Can you work these out from the model? Positions are in its coordinate system, mm. Face numbers are marked on the shaded views. A direction names the side the tool comes from. Round coordinates to 2 decimals unless told otherwise and drop trailing zeros. Order: outer loops, then holes, each group sorted by start corner. A loop starts at its lowest first (then second) coordinate and runs counter-clockwise, first axis right, second up.
Q1. If we section it at A-A (z = 17.75): Please give me the cut outline in (x, y) (3 decimals).
Q2. Will these pins go through, and if not, where does the flat tip stop? P1, Ø2, axis at x = 3, y = -6, coming from the +Z side; P2, Ø1.6, axis at x = 6, z = 19.5, coming from the -Y side; P3, Ø6, axis at x = -2, y = 1, coming from the +Z side.
Q3. We'd pull the mould along Y, two halves only. Please class the marked faces 4, 5 and 6: pulls with the +Y half, pulls with the -Y half, needs draft (parallel to the pull), parting line crosses it, or undercut.
Q4. If I drill on line 1 (Y direction, x = 0, z = 7.75) (3 decimals); line 2 (Z direction, x = 4.5, y = -5.75); line 3 (Y direction, x = -3.75, z = 5.25), over which ranges is the centre line in solid material (lowest first)?
Q5. For the marked faces 1, 2 and 3, which set-ups out of +Z, -Z, +X, -X, +Y, -Y let a thin tool reach every point of the face, with its end or its side?
Q6. If we section it at C-C (x = 6.5): Please give me the cut outline in (y, z).
Q7. If we section it at D-D (y = -2.75): Please give me the cut outline in (x, z) (3 decimals).
Q8. If we section it at B-B (z = 11.5): Please give me the cut outline in (x, y) (1 decimal), plus the area to 3 significant figures.
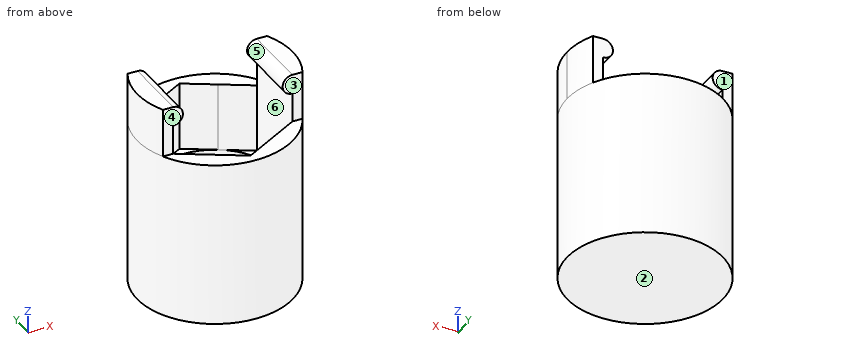
from build123d import *

# Parameters (mm, degrees)
F0_R      = 6.125
F1_DEPTH  = 2
F0_R_2    = 8
F2_DEPTH  = 10
F3_R      = 8
F4_DEPTH  = 7
F6_DEPTH  = 5
F8_DEPTH  = 7.0725407976
F10_DEPTH = 7.0725407976


with BuildPart() as f1:
    # F0 (on Top) → F1 (new body)
    with BuildSketch(Plane.XY):
        Circle(F0_R)
    extrude(amount=F1_DEPTH)

    # F0 (on Top) → F2 (join)
    with BuildSketch(Plane.XY):
        Circle(F0_R_2)
        Circle(F0_R, mode=Mode.SUBTRACT)
    extrude(amount=F2_DEPTH)

    # F3 (on face) → F4 (join)
    with BuildSketch(Plane.XY.offset(10)):
        Circle(F3_R)
        Polygon((3.0624998551, 5.3044056818), (6.125, 3.5362703988), (6.125, 0), (6.125, -3.5362703988), (3.0625000444, -5.3044055725), (0, -7.0725407976), (-3.0625000444, -5.3044055725), (-6.125, -3.5362703988), (-6.125, 0), (-6.125, 3.5362703988), (-3.0624999859, 5.3044056063), (0, 7.0725407976), align=None, mode=Mode.SUBTRACT)
    extrude(amount=F4_DEPTH)

    # F5 (on face) → F6 (join)
    with BuildSketch(Plane.XY.offset(17)):
        with BuildLine():
            Line((-6.125, -3.5362703988), (-6.125, 3.5362703988))
            Line((-6.125, 3.5362703988), (-7.1759871563, 3.5362703988))
            ThreePointArc((-7.1759871563, 3.5362703988), (-8, 0), (-7.1759871563, -3.5362703988))
            Line((-7.1759871563, -3.5362703988), (-6.125, -3.5362703988))
        make_face()
        with BuildLine():
            ThreePointArc((8, 0), (7.7912738769, 1.8155030639), (7.1759871563, 3.5362703988))
            Line((7.1759871563, 3.5362703988), (6.125, 3.5362703988))
            Line((6.125, 3.5362703988), (6.125, -3.5362703988))
            Line((6.125, -3.5362703988), (7.1759871563, -3.5362703988))
            ThreePointArc((7.1759871563, -3.5362703988), (7.7912738769, -1.8155030639), (8, 0))
        make_face()
    extrude(amount=F6_DEPTH)

    # F7 (on face) → F8 (join, through all)
    with BuildSketch(Plane(origin=(0, 3.5362703988, 0), x_dir=(-1, 0, 0), z_dir=(0, 1, 0))):
        with BuildLine():
            Line((6.125, 20), (6.125, 22))
            ThreePointArc((6.125, 22), (5.125, 21), (6.125, 20))
        make_face()
    extrude(amount=-F8_DEPTH)

    # F9 (on face) → F10 (join, through all)
    with BuildSketch(Plane(origin=(0, 3.5362703988, 0), x_dir=(-1, 0, 0), z_dir=(0, 1, 0))):
        with BuildLine():
            Line((-6.125, 22), (-6.125, 20))
            ThreePointArc((-6.125, 20), (-5.125, 21), (-6.125, 22))
        make_face()
    extrude(amount=-F10_DEPTH)


solid = f1.part
Solution:
1. outline: (-7.176, -3.536) - (-6.125, -3.536) - (-6.125, 3.536) - (-7.176, 3.536) arc R8 ccw to start; (6.125, -3.536) - (7.176, -3.536) arc R8 ccw to (7.176, 3.536) - (6.125, 3.536) - close
2. P1: stops at z = 17
2. P2: stops at y = -3.54
2. P3: stops at z = 2
3. face 4: pulls with the -Y half
3. face 5: needs draft
3. face 6: undercut
4. line 1: y = -8 to -6.125, 6.125 to 8
4. line 2: z = 0 to 17
4. line 3: y = -7.07 to -4.84, 4.84 to 7.07
5. face 1: +Z, +X, -X, +Y
5. face 2: -Z, +X, -X, +Y, -Y
5. face 3: +Z, +X, -X, -Y
6. outline: (-4.66, 0) - (4.66, 0) - (4.66, 17) - (3.54, 17) - (3.54, 22) - (-3.54, 22) - (-3.54, 17) - (-4.66, 17) - close
7. outline: (-7.512, 0) - (7.512, 0) - (7.512, 22) - (6.125, 22) arc R1 ccw to (6.125, 20) - (6.125, 10) - (5.473, 10) - (5.473, 2) - (-5.473, 2) - (-5.473, 10) - (-6.125, 10) - (-6.125, 20) arc R1 ccw to (-6.125, 22) - (-7.512, 22) - close
8. outline: circle Ø16 at (0, 0); hole (-6.1, -3.5) - (0, -7.1) - (6.1, -3.5) - (6.1, 3.5) - (0, 7.1) - (-6.1, 3.5) - close
8. area: 71.1 mm2
